from build123d import *

# Parameters (mm, degrees)
SKETCH1_W           = 323.85
SKETCH1_H           = 457.2
BOSS_EXTRUDE1_DEPTH = 4.3434
SKETCH2_W           = 271.78
SKETCH2_H           = 273.05
CUT_EXTRUDE1_DEPTH  = 5.3434
FILLET1_R           = 7.14375
SKETCH4_W           = 88.9
SKETCH4_H           = 184.911324328
CUT_EXTRUDE3_DEPTH  = 5.3434
FILLET2_R           = 7.14375


with BuildPart() as part:
    # Sketch1 → Boss-Extrude1 (new body)
    with BuildSketch(Plane.XY):
        Rectangle(SKETCH1_W, SKETCH1_H)
    extrude(amount=BOSS_EXTRUDE1_DEPTH)

    # Sketch2 → Cut-Extrude1 (cut, through all)
    with BuildSketch(Plane.XY.offset(4.3434)):
        with Locations((0, -68.707)):
            Rectangle(SKETCH2_W, SKETCH2_H)
    extrude(amount=-CUT_EXTRUDE1_DEPTH, mode=Mode.SUBTRACT)

    # Fillet1
    fillet1_edges = [part.edges().sort_by_distance(p)[0] for p in [
        (135.89, 67.818, 2.1717),
        (135.89, -205.232, 2.1717),
        (-135.89, -205.232, 2.1717),
        (-135.89, 67.818, 2.1717),
        (161.925, -228.6, 2.1717),
        (-161.925, -228.6, 2.1717),
        (-161.925, 228.6, 2.1717),
        (161.925, 228.6, 2.1717),
    ]]
    fillet(fillet1_edges, radius=FILLET1_R)

    # Sketch4 → Cut-Extrude3 (cut, through all)
    with BuildSketch(Plane.XY.offset(4.3434)):
        with Locations((-91.44, 131.800937836)):
            Rectangle(SKETCH4_W, SKETCH4_H)
    extrude(amount=-CUT_EXTRUDE3_DEPTH, mode=Mode.SUBTRACT)

    # Fillet2
    fillet2_edges = [part.edges().sort_by_distance(p)[0] for p in [
        (-46.99, 67.818, 2.1717),
        (-46.99, 224.2566, 2.1717),
        (-135.89, 224.2566, 2.1717),
    ]]
    fillet(fillet2_edges, radius=FILLET2_R)


solid = part.part
Read the model definition and answer for the solid it produces. Units are mm, in the model's axes. Round coordinates to 2 decimals unless told otherwise and drop trailing zeros. Loops run counter-clockwise (first coordinate to the right, second up) from the corner with the lowest first, then second, coordinate; pieces in that order, holes last. Notation, with made-up numbers: (73.5, -35) - (116.5, -35) arc R28 cw to (116.5, -17) - close; hole circle Ø1 at (14, -16.75). An arc over 180 degrees is marked (long way). One line per question, with ' | ' between items. Start each with the question number.
Q1. Section B-B on y = 43.5 is taken. Give the vertices of the cut face in (x, z) (3 decimals).
Q2. Section C-C on z = 2.3 is taken. Give the vertices of the cut face in (x, y) (1 decimal).
Q3. Section A-A on x = -68.5 is taken. Give the vertices of the cut face in (y, z).
Q4. Find the intervals of material crossed by L1, parallel to Y at x = -79, z = 3.45; L2, parallel to Y at x = 93.5, z = 1.5; L3, parallel to X at y = 13.5, z = 2.1 (3 decimals), in increasing order.
Established:
1) outline: (-161.925, 0) - (-135.89, 0) - (-135.89, 4.343) - (-161.925, 4.343) - close; (135.89, 0) - (161.925, 0) - (161.925, 4.343) - (135.89, 4.343) - close
2) outline: (-161.9, -221.5) arc R7.1 ccw to (-154.8, -228.6) - (154.8, -228.6) arc R7.1 ccw to (161.9, -221.5) - (161.9, 221.5) arc R7.1 ccw to (154.8, 228.6) - (-154.8, 228.6) arc R7.1 ccw to (-161.9, 221.5) - close; hole (-135.9, -198.1) arc R7.1 ccw to (-128.7, -205.2) - (128.7, -205.2) arc R7.1 ccw to (135.9, -198.1) - (135.9, 60.7) arc R7.1 ccw to (128.7, 67.8) - (-39.8, 67.8) arc R7.1 cw to (-47, 75) - (-47, 217.1) arc R7.1 ccw to (-54.1, 224.3) - (-128.7, 224.3) arc R7.1 ccw to (-135.9, 217.1) - close
3) outline: (-228.6, 0) - (-205.23, 0) - (-205.23, 4.34) - (-228.6, 4.34) - close; (224.26, 0) - (228.6, 0) - (228.6, 4.34) - (224.26, 4.34) - close
4) L1: -228.6 to -205.23, 224.26 to 228.6 | L2: -228.6 to -205.23, 67.82 to 228.6 | L3: -161.925 to -135.89, 135.89 to 161.925
